Study the drawing (mm; zero at the part's minimum x, y, z) and answer. A direction names the side the tool comes from. Round coordinates to 2 decimals unless told otherwise and drop trailing zeros. Write each loop counter-clockwise with the first axis right and the second up, starting at its lowest first coordinate (ties: lowest second). Pieces come first, ordered by that corner, then holes.
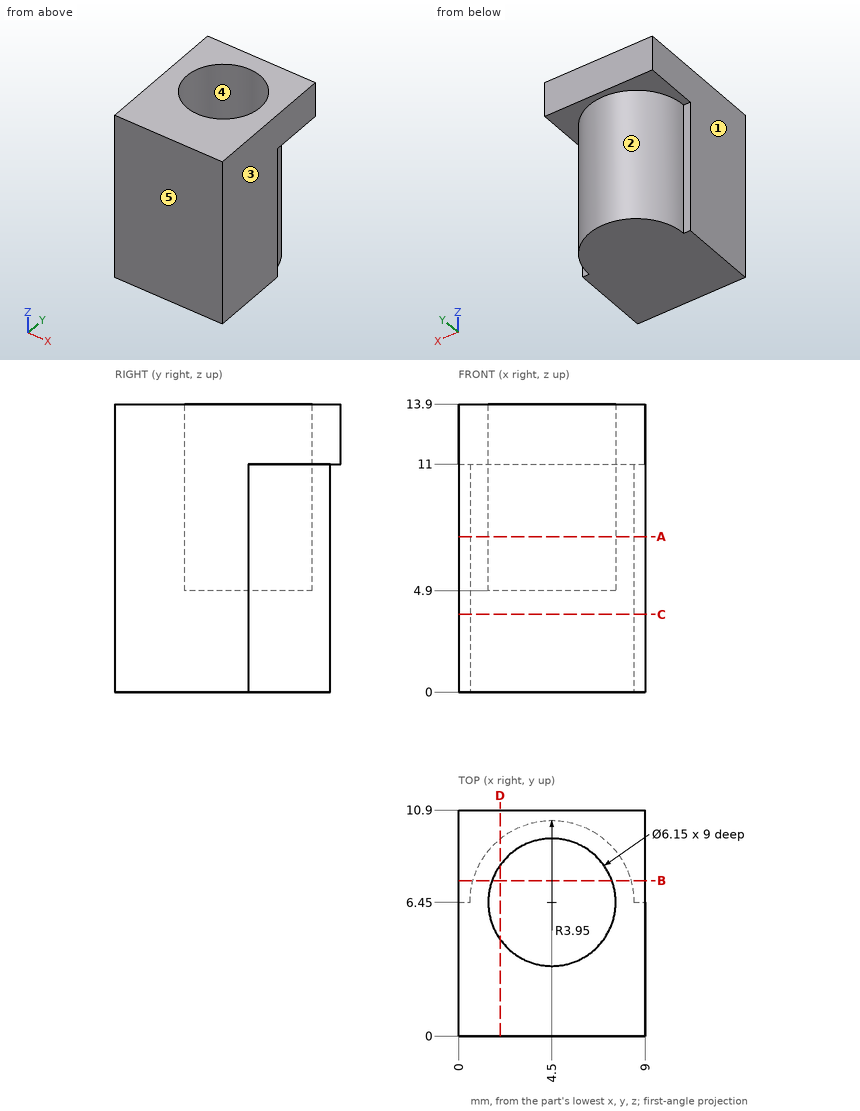
1. Section A-A on z = 7.5 is taken. Determine the outline of the cut face in (x, y) (3 decimals).
Geometry says:
outline: (0, 0) - (9, 0) - (9, 6.45) - (8.45, 6.45) arc R3.95 ccw to (0.55, 6.45) - (0, 6.45) - close; hole circle Ø6.15 at (4.5, 6.45)
2. Section D-D on x = 2 is taken. Determine the outline of the cut face in (y, z).
Geometry says:
outline: (0, 0) - (9.51, 0) - (9.51, 11) - (10.9, 11) - (10.9, 13.9) - (8.24, 13.9) - (8.24, 4.9) - (4.66, 4.9) - (4.66, 13.9) - (0, 13.9) - close
3. A tool of negligible diameter and unlimited length cuts with its end or side. For the marked faces 1 and 2, from which of +Z, -Z, +X, -X, +Y, -Y can it reach the whole face along a straight path? Write none if from no direction.
Geometry says:
face 1: +Z, -Z, -X, +Y, -Y
face 2: -Z, +Y
4. Given pin 1 (1.8 mm diameter, centred on x = 3.5, y = 5, fed in from +Z), flat-ended and moving along its own axis, determine where the tip first touches the part or whether it passes through.
Geometry says:
pin 1: stops at z = 4.9
5. Straight lines are drawn through the part: line 1 along Y through (x, z) = (4.5, 7.25) (3 decimals); line 2 along Y through (x, z) = (4.5, 12) (3 decimals); line 3 along Z through (x, y) = (4.5, 8.25). For each, find the intervals that lie inside material, in ascending order.
Geometry says:
line 1: y = 0 to 3.375, 9.525 to 10.4
line 2: y = 0 to 3.375, 9.525 to 10.9
line 3: z = 0 to 4.9
6. Section B-B on y = 7.5 is taken. Determine the outline of the cut face in (x, z).
Geometry says:
outline: (0, 11) - (0.69, 11) - (0.69, 0) - (8.31, 0) - (8.31, 11) - (9, 11) - (9, 13.9) - (7.39, 13.9) - (7.39, 4.9) - (1.61, 4.9) - (1.61, 13.9) - (0, 13.9) - close
7. Section C-C on z = 3.75 is taken. Determine the outline of the cut face in (x, y), plus the area to 3 significant figures.
Geometry says:
outline: (0, 0) - (9, 0) - (9, 6.45) - (8.45, 6.45) arc R3.95 ccw to (0.55, 6.45) - (0, 6.45) - close
area: 82.6 mm2
8. For a pull along X with two mould halves and no side action, classify the marked faces 3, 4 and 5 as released by +X, released by -X, zero draft, split by the parting line, or undercut.
Geometry says:
face 3: released by +X
face 4: undercut
face 5: zero draft
